The listing builds one solid part. Answer for the finished solid, in the listing's coordinates (mm). Give positions to 0.01 mm unless a question says otherwise; leave off trailing zeros. One line per question, with ' | ' between items. Start each with the question number.
from build123d import *

# Parameters (mm, degrees)
F0_W           = 304.8
F0_H           = 6.35
F1_DEPTH       = 38.1
F3_D           = 2.7051
F3_DEPTH       = 15.08125
F3_TIP         = 0.8126940303
F5_D           = 3.2639
F5_CSINK_D     = 6.477
F5_CSINK_ANGLE = 82
F7_D           = 3.7973
F7_CSINK_D     = 7.7978
F7_CSINK_ANGLE = 82


with BuildPart() as f1:
    # F0 (on Top) → F1 (new body)
    with BuildSketch(Plane.XY):
        Rectangle(F0_W, F0_H)
    extrude(amount=F1_DEPTH)

    # F3
    with Locations(Plane(origin=(0, 0, 0), x_dir=(1, 0, 0), z_dir=(0, 0, -1))):
        with Locations((-127, 0), (127, 0), (0, 0)):
            Hole(F3_D / 2, depth=F3_DEPTH)
            with Locations((0, 0, -(F3_DEPTH + F3_TIP / 2))):  # 118° drill point
                Cone(0, F3_D / 2, F3_TIP, mode=Mode.SUBTRACT)

    # F5 (through all)
    with Locations(Plane(origin=(0, 3.175, 0), x_dir=(-1, 0, 0), z_dir=(0, 1, 0))):
        with Locations((149.225, 31.75), (149.225, 6.35), (-149.225, 31.75), (-149.225, 6.35)):
            CounterSinkHole(F5_D / 2, F5_CSINK_D / 2, counter_sink_angle=F5_CSINK_ANGLE)

    # F7 (through all)
    with Locations(Plane(origin=(0, 3.175, 0), x_dir=(-1, 0, 0), z_dir=(0, 1, 0))):
        with Locations((-85.725, 3.81), (22.225, 3.81), (53.975, 3.81), (111.125, 3.81), (-85.725, 16.51), (22.225, 16.51)):
            CounterSinkHole(F7_D / 2, F7_CSINK_D / 2, counter_sink_angle=F7_CSINK_ANGLE)


solid = f1.part
1. Straight lines are drawn through the part: L1, parallel to X at y = -1.9, z = 3.81; L2, parallel to Z at x = -23, y = 2; L3, parallel to Z at x = -112.5, y = 2. For each, find the intervals that lie inside material, in ascending order.
2. Determine the mould class of faces 1 (the conical face through (-24.22, 0.99, 3.9)), 2 (the flat face through (152.4, 0, 19)), 3 (the flat face through (-2, 0, 38.1)) for opening direction X: released by +X, released by -X, zero draft, split by the parting line, or undercut.
3. Each of these flat-tipped pins is pushed along its axis until it touches: pin 1 Ø5 at (x, z) = (85.725, 16.51) entering from +Y; pin 2 Ø4.5 at (x, z) = (-22.225, 16.51) entering from +Y; pin 3 Ø6 at (x, z) = (85.725, 3.81) entering from +Y. Where does it stop, or does it pass through?
Check sheet entries:
1) L1: x = -152.4 to -113.02, -109.23 to -55.87, -52.08 to -24.12, -20.33 to 83.83, 87.62 to 152.4 | L2: z = 0 to 1.04, 6.58 to 13.74, 19.28 to 38.1 | L3: z = 0 to 1.28, 6.34 to 38.1
2) face 1: undercut | face 2: released by +X | face 3: zero draft
3) pin 1: stops at y = 1.57 | pin 2: stops at y = 1.28 | pin 3: stops at y = 2.14
